Here's how the part is built. I have some questions about the finished solid (model axes, mm). Coordinates: 2 decimals unless noted, no trailing zeros. Loops run counter-clockwise (first coordinate to the right, second up) from the corner with the lowest first, then second, coordinate; pieces in that order, holes last.
```python
from build123d import *

# Parameters (mm, degrees)
SKETCH2_W           = 80
SKETCH2_H           = 12.7
BOSS_EXTRUDE1_DEPTH = 12.7
SKETCH3_R           = 2
CUT_EXTRUDE1_DEPTH  = 43.445406112
SKETCH4_RX          = 8.89
SKETCH4_RY          = 4.6609
CUT_EXTRUDE3_DEPTH  = 44.847234804


with BuildPart() as part:
    # Sketch2 → Boss-Extrude1 (new body)
    with BuildSketch(Plane(origin=(0, 0, 0), x_dir=(1, 0, 0), z_dir=(0, 1, 0))):
        Rectangle(SKETCH2_W, SKETCH2_H)
    extrude(amount=BOSS_EXTRUDE1_DEPTH)

    # Sketch3 → Cut-Extrude1 (cut, through all)
    with BuildSketch(Plane(origin=(0, 12.7, 0), x_dir=(1, 0, 0), z_dir=(0, 1, 0))):
        with Locations(Location((-35, 0, 0), (0, 0, 270))):
            Circle(SKETCH3_R)
        with Locations(Location((-20, 0, 0), (0, 0, 270))):
            Circle(SKETCH3_R)
        with Locations(Location((35, 0, 0), (0, 0, 270))):
            Circle(SKETCH3_R)
        with Locations(Location((20, 0, 0), (0, 0, 270))):
            Circle(SKETCH3_R)
    extrude(amount=-CUT_EXTRUDE1_DEPTH, mode=Mode.SUBTRACT)

    # Sketch4 → Cut-Extrude3 (cut, through all)
    with BuildSketch(Plane.XY.offset(6.35)):
        with Locations((0, 6.20775407)):
            Ellipse(SKETCH4_RX, SKETCH4_RY)
    extrude(amount=-CUT_EXTRUDE3_DEPTH, mode=Mode.SUBTRACT)


solid = part.part
```
1. I need wall thicknesses on line 1 along X through (y, z) = (6, -2.25); line 2 along X through (y, z) = (3, 0); line 3 along X through (y, z) = (5.75, 0). Which ranges of each line are inside material? Lowest first, please.
2. For pin 1 (3 mm diameter, centred on x = -20, z = 0, fed in from +Y), with a flat end and sliding along its axis, tell me the tip position at first contact or that it passes through.
3. We'd pull the mould along Z, two halves only. Please class faces 1 (the cylindrical face through (-37, 6, 0)), 2 (the flat face through (-1, 12.7, 0)), 3 (the flat face through (-1, 12, -6.35)), 4 (the cylindrical face through (22, 6, 0)): +Z half, -Z half, draft (parallel to the pull), parting line (faces both ways), or undercut.
4. I want a section at A-A (x = 35). Please give me the cut outline in (y, z), then the cut area to 3 significant figures.
5. I want a section at B-B (z = 0.5). Give the number of separate pieces and of enclosed holes in the cut face, then the cut area to 3 significant figures.
Response values:
1. line 1: x = -40 to -8.88, 8.88 to 40
1. line 2: x = -40 to -37, -33 to -22, -18 to -6.45, 6.45 to 18, 22 to 33, 37 to 40
1. line 3: x = -40 to -37, -33 to -22, -18 to -8.85, 8.85 to 18, 22 to 33, 37 to 40
2. pin 1: passes through
3. face 1: undercut
3. face 2: draft
3. face 3: -Z half
3. face 4: undercut
4. outline: (0, -6.35) - (12.7, -6.35) - (12.7, -2) - (0, -2) - close; (0, 2) - (12.7, 2) - (12.7, 6.35) - (0, 6.35) - close
4. area: 110 mm2
5. separate pieces: 5
5. enclosed holes: 1
5. area: 689 mm2
